Input: part model. Units: mm. Frame: model coordinates. A direction names the side the tool comes from. Round coordinates to 2 decimals unless told otherwise and drop trailing zeros. Loops run counter-clockwise (first coordinate to the right, second up) from the corner with the lowest first, then second, coordinate; pieces in that order, holes last. Notation, with made-up numbers: (-34, 21) -> (-22, 21) arc R23 cw to (-22, 32) -> close; hole circle Ø1 at (70, 79). An arc over 180 degrees is marked (long way). Answer in a Markdown table with one row per item. Add a question column.
Q1. Ray query, L1, parallel to Y at x = 0, z = 11; L2, parallel to Y at x = 0, z = 40; L3, parallel to Z at x = 30.5, y = 4. Return the intervals inside material, ascending. Write a range as from..to.
Q2. Section B-B, the plane x = 0. Output: boundary loops of the cut face in (y, z), and give its area (3 significant figures).
Q3. Reachability of faces 1 (the face through (-29.3, 0.6, 33.02)), 2 (the face through (-1, -42.572, 16)) from +Z, -Z, +X, -X, +Y, -Y: full face, straight path, thin tool, end or side. Return the list, or none.
Q4. Section D-D, the plane y = -27. Output: boundary loops of the cut face in (x, z), and give its area (3 significant figures).
Q5. Section C-C, the plane z = 37. Output: boundary loops of the cut face in (x, y), and give its area (3 significant figures).
Q6. Section A-A, the plane y = 0. Output: boundary loops of the cut face in (x, z).
Q7. Pin query (flat end, axial travel): pin 1 (6 mm diameter, centred on x = 13, y = -5, fed in from -Z); pin 2 (1 mm diameter, centred on x = -24, z = 38, fed in from +Y); pin 3 (2 mm diameter, centred on y = 14, z = 43, fed in from +X); pin 4 (6 mm diameter, centred on x = 26, y = -31, fed in from +Z). Return the tip coordinate at first contact, or that it passes through.
```python
from build123d import *

# Parameters (mm, degrees)
F0_W      = 86.230226
F0_H      = 85.144274
F1_DEPTH  = 33.02
F2_R      = 28.889637
F2_R_2    = 17.278363
F3_DEPTH  = 25.4
F3_FACE_R = 17.278363
F4_DEPTH  = 127


with BuildPart() as f1:
    # F0 (on Top) → F1 (new body)
    with BuildSketch(Plane.XY):
        Rectangle(F0_W, F0_H)
    extrude(amount=F1_DEPTH)

    # F2 (on face) → F3 (join)
    with BuildSketch(Plane.XY.offset(33.02)):
        Circle(F2_R)
        Circle(F2_R_2, mode=Mode.SUBTRACT)
    extrude(amount=F3_DEPTH)

    # F3_face (on face) → F4 (cut)
    with BuildSketch(Plane.XY.offset(33.02)):
        Circle(F3_FACE_R)
    extrude(amount=-F4_DEPTH, mode=Mode.SUBTRACT)


solid = f1.part
```
Answer block:
| question | item | result |
|---|---|---|
| 1 | L1 | -42.57..-17.28, 17.28..42.57 |
| 1 | L2 | -28.89..-17.28, 17.28..28.89 |
| 1 | L3 | 0..33.02 |
| 2 | outline | (-42.57, 0) -> (-17.28, 0) -> (-17.28, 58.42) -> (-28.89, 58.42) -> (-28.89, 33.02) -> (-42.57, 33.02) -> close; (17.28, 0) -> (42.57, 0) -> (42.57, 33.02) -> (28.89, 33.02) -> (28.89, 58.42) -> (17.28, 58.42) -> close |
| 2 | area | 2,260 mm^2 |
| 3 | face 1 | +Z |
| 3 | face 2 | +Z, -Z, +X, -X, -Y |
| 4 | outline | (-43.12, 0) -> (43.12, 0) -> (43.12, 33.02) -> (10.28, 33.02) -> (10.28, 58.42) -> (-10.28, 58.42) -> (-10.28, 33.02) -> (-43.12, 33.02) -> close |
| 4 | area | 3,370 mm^2 |
| 5 | outline | circle Ø57.78 at (0, 0); hole circle Ø34.56 at (0, 0) |
| 5 | area | 1,680 mm^2 |
| 6 | outline | (-43.12, 0) -> (-17.28, 0) -> (-17.28, 58.42) -> (-28.89, 58.42) -> (-28.89, 33.02) -> (-43.12, 33.02) -> close; (17.28, 0) -> (43.12, 0) -> (43.12, 33.02) -> (28.89, 33.02) -> (28.89, 58.42) -> (17.28, 58.42) -> close |
| 7 | pin 1 | through |
| 7 | pin 2 | y = 16.8 |
| 7 | pin 3 | x = 25.8 |
| 7 | pin 4 | z = 33.02 |
